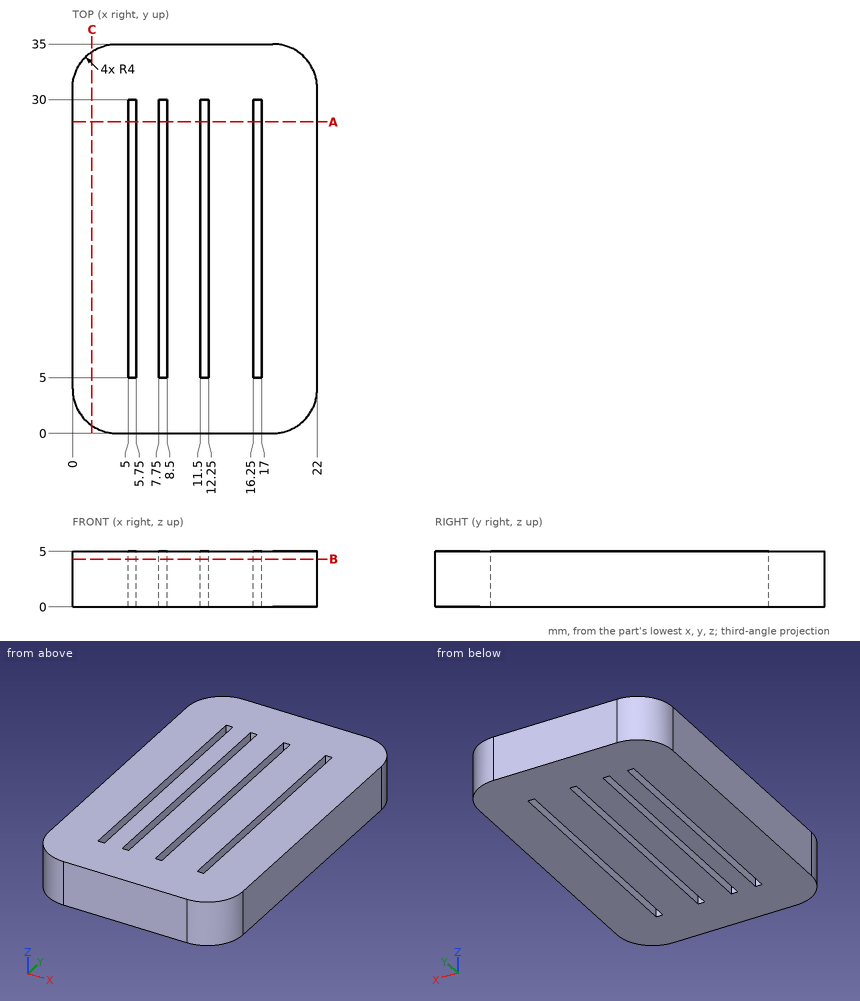
Source: three-view drawing plus pictorial views. Frame: mm from the lowest corner of the part. Give positions to 0.01 mm unless a question says otherwise; leave off trailing zeros. Write each loop counter-clockwise with the first axis right and the second up, starting at its lowest first coordinate (ties: lowest second). Pieces come first, ordered by that corner, then holes. Notation, with made-up numbers: M -34.5,1 L 11.5,1 A14 ccw 11.5,15 Z; hole C -31,4 d3. An arc over 180 degrees is marked long. Use one line per item in the form item = value.
1. Cut plane B-B on z = 4.3. Return loops of the section in (x, y).
Outcome:
outline = M 0,4 A4 ccw 4,0 L 18,0 A4 ccw 22,4 L 22,31 A4 ccw 18,35 L 4,35 A4 ccw 0,31 Z; hole M 5,5 L 5.75,5 L 5.75,30 L 5,30 Z; hole M 7.75,5 L 8.5,5 L 8.5,30 L 7.75,30 Z; hole M 11.5,5 L 12.25,5 L 12.25,30 L 11.5,30 Z; hole M 16.25,5 L 17,5 L 17,30 L 16.25,30 Z
2. Cut plane A-A on y = 28. Return loops of the section in (x, z), and give its area (3 significant figures).
Outcome:
outline = M 0,0 L 5,0 L 5,5 L 0,5 Z; M 5.75,0 L 7.75,0 L 7.75,5 L 5.75,5 Z; M 8.5,0 L 11.5,0 L 11.5,5 L 8.5,5 Z; M 12.25,0 L 16.25,0 L 16.25,5 L 12.25,5 Z; M 17,0 L 22,0 L 22,5 L 17,5 Z
area = 95.0 mm²
3. Ray query, L1, parallel to X at y = 22, z = 4.1; L2, parallel to Y at x = 5.25, z = 1.55; L3, parallel to X at y = 33.5, z = 4.2. Return the intervals inside material, ascending.
Outcome:
L1 = 0 to 5, 5.75 to 7.75, 8.5 to 11.5, 12.25 to 16.25, 17 to 22
L2 = 0 to 5, 30 to 35
L3 = 0.88 to 21.12
4. Cut plane C-C on x = 1.75. Return loops of the section in (y, z), and give its area (3 significant figures).
Outcome:
outline = M 0.69,0 L 34.31,0 L 34.31,5 L 0.69,5 Z
area = 168 mm²
